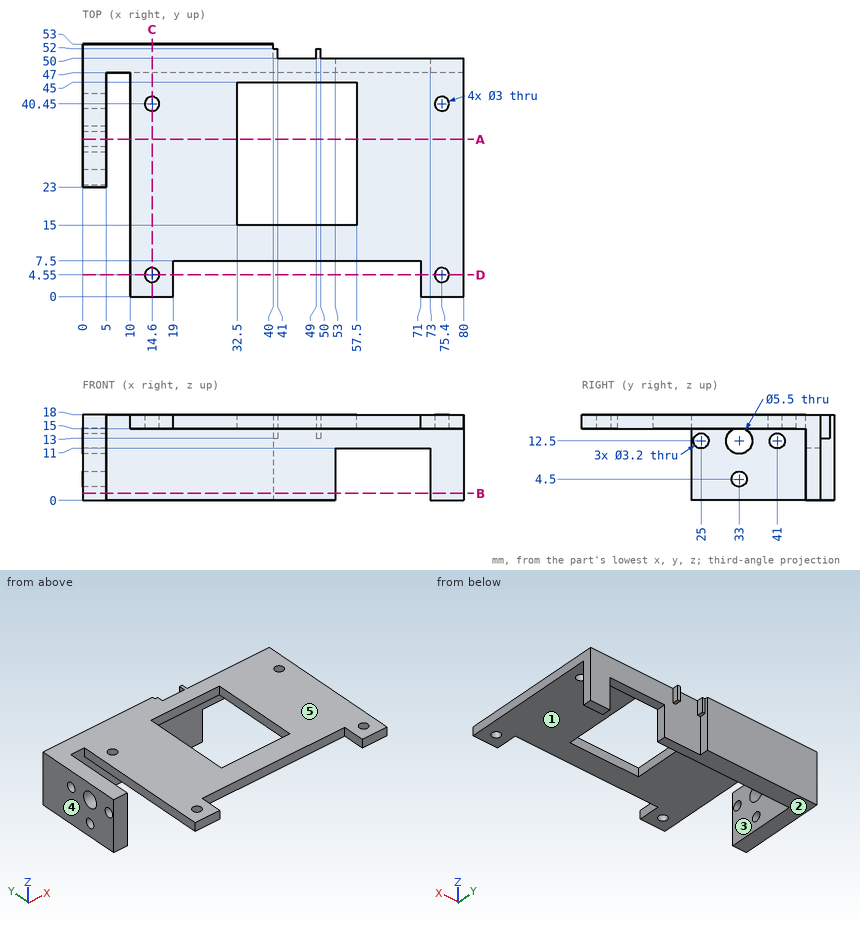
The figure shows three views and two pictorial views of one solid part (mm, origin at its lowest corner). Answer the questions. A direction names the side the tool comes from. Coordinates: 2 decimals unless noted, no trailing zeros. Loops run counter-clockwise (first coordinate to the right, second up) from the corner with the lowest first, then second, coordinate; pieces in that order, holes last. Notation, with made-up numbers: M 51,7 L 88,7 A10 cw 88,14 Z; hole C 35,-38.5 d8. An arc over 180 degrees is marked long. Use CSV: the item, a comma, the result in double quotes. Start each with the question number.
(1) Find section C-C, the plane x = 14.6. Give the vertices of the cut face in (y, z), then the cut area to 3 significant figures.
(2) Find section A-A, the plane y = 33. Give the vertices of the cut face in (x, z), then the cut area to 4 significant figures.
(3) Given pin 1 Ø12 at (x, y) = (14.5, 12) entering from -Z; pin 2 Ø1.5 at (y, z) = (51, 13) entering from +X; pin 3 Ø10 at (x, z) = (36.5, 13) entering from -Y; pin 4 Ø6 at (x, y) = (41, 39.5) entering from -Z, each flat-ended and moving along its own axis, determine where each tip first touches the part or whether it passes through.
(4) For a pull along X with two mould halves and no side action, classify the marked faces 3, 4 and 5 as +X half, -X half, draft (parallel to the pull), parting line (faces both ways), or undercut.
(5) Find section B-B, the plane z = 1.5. Give the vertices of the cut face in (x, y), then the cut area to 3 significant figures.
(6) Find section D-D, the plane y = 4.55. Give the vertices of the cut face in (x, z).
(7) For the marked faces 1 and 2, determine the directions among +Z, -Z, +X, -X, +Y, -Y from which every point of the face is accessible in a straight line to the end or side of a thin tool.
(8) Consider line 1 (Y direction, x = 3.75, z = 12.5); line 2 (X direction, y = 40.45, z = 17.4); line 3 (Y direction, x = 75.4, z = 16.65). Determine where each line is inside the solid, lowest interval first.
Recorded:
1,outline,"M 0,15 L 3.05,15 L 3.05,18 L 0,18 Z; M 6.05,15 L 38.95,15 L 38.95,18 L 6.05,18 Z; M 41.95,15 L 47,15 L 47,0 L 53,0 L 53,18 L 41.95,18 Z"
1,area,"231 mm^2"
2,outline,"M 0,0 L 5,0 L 5,2.9 L 0,2.9 Z; M 0,6.1 L 5,6.1 L 5,9.75 L 0,9.75 Z; M 0,15.25 L 5,15.25 L 5,18 L 0,18 Z; M 10,15 L 32.5,15 L 32.5,18 L 10,18 Z; M 57.5,15 L 80,15 L 80,18 L 57.5,18 Z"
2,area,"181.5 mm^2"
3,pin 1,"stops at z = 15"
3,pin 2,"stops at x = 50"
3,pin 3,"stops at y = 7.5"
3,pin 4,"passes through"
4,face 3,"undercut"
4,face 4,"-X half"
4,face 5,"draft"
5,outline,"M 0,23 L 5,23 L 5,47 L 53,47 L 53,50 L 40,50 L 40,53 L 0,53 Z; M 73,47 L 80,47 L 80,50 L 73,50 Z"
5,area,"420 mm^2"
6,outline,"M 10,15 L 13.1,15 L 13.1,18 L 10,18 Z; M 16.1,15 L 19,15 L 19,18 L 16.1,18 Z; M 71,15 L 73.9,15 L 73.9,18 L 71,18 Z; M 76.9,15 L 80,15 L 80,18 L 76.9,18 Z"
7,face 1,"-Z, +X, -Y"
7,face 2,"-Z, +X, -X, +Y, -Y"
8,line 1,"y = 23 to 23.4, 26.6 to 30.25, 35.75 to 39.4, 42.6 to 53"
8,line 2,"x = 0 to 5, 10 to 13.1, 16.1 to 32.5, 57.5 to 73.9, 76.9 to 80"
8,line 3,"y = 0 to 3.05, 6.05 to 38.95, 41.95 to 50"
